Can you work these out from the model? Positions are in its coordinate system, mm. Face numbers are marked on the shaded views. A direction names the side the tool comes from. Give positions to 0.01 mm unless a question says otherwise; leave off trailing zeros. Loops run counter-clockwise (first coordinate to the right, second up) from the corner with the lowest first, then second, coordinate; pieces in that order, holes last. Notation, with made-up numbers: (-33.5, 79) -> (-11.5, 79) arc R30 ccw to (-11.5, 102) -> close; hole circle Ø9 at (63.5, 49). An arc over 180 degrees is marked (long way). One line per question, with ' | ' between items.
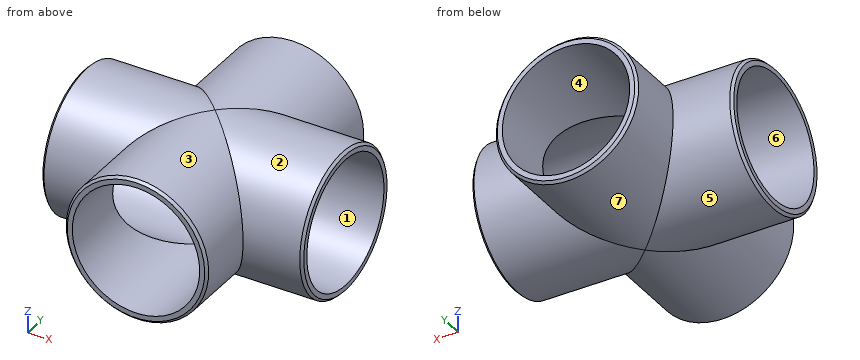
from build123d import *

# Parameters (mm, degrees)
RUNROUTE_R             = 57.15
RUNEXTRUDE_DEPTH       = 104.648
OUTLETROUTE_R          = 57.15
OUTLETEXTRUDE_DEPTH    = 104.648
CROSSSHELL_START       = -104.648
CROSSSHELL_OUTLINE_R   = 51.1302
CROSSSHELL_DEPTH       = 209.296
CROSSSHELL_2_OUTLINE_R = 51.1302
CROSSSHELL_2_DEPTH     = 209.296
CROSSCHAMFER_SIZE      = 2.0066


with BuildPart() as part:
    # RunRoute → RunExtrude (new body)
    with BuildSketch(Plane(origin=(0, 0, 0), x_dir=(0, 0, -1), z_dir=(1, 0, 0))):
        Circle(RUNROUTE_R)
    runextrude = extrude(amount=RUNEXTRUDE_DEPTH)

    # RunExtrudeMirror: RunExtrude across plane
    add(runextrude.mirror(Plane(origin=(0, 0, 0), x_dir=(0, 0, 1), z_dir=(1, 0, 0))))

    # OutletRoute → OutletExtrude (add)
    with BuildSketch(Plane(origin=(0, 0, 0), x_dir=(1, 0, 0), z_dir=(0, 1, 0))):
        with Locations(Location((0, 0, 0), (0, 0, 270))):
            Circle(OUTLETROUTE_R)
    outletextrude = extrude(amount=OUTLETEXTRUDE_DEPTH)

    # OutletExtrudeMirror: OutletExtrude across plane
    add(outletextrude.mirror(Plane.ZX))

    # CrossShell: read off the stored shape, not the designer's step
    # CrossShell outline → CrossShell (cut)
    with BuildSketch(Plane.YZ.offset(CROSSSHELL_START)):
        Circle(CROSSSHELL_OUTLINE_R)
    extrude(amount=CROSSSHELL_DEPTH, mode=Mode.SUBTRACT)

    # CrossShell 2 outline → CrossShell 2 (cut)
    with BuildSketch(Plane(origin=(0, 0, 0), x_dir=(1, 0, 0), z_dir=(0, 1, 0)).offset(CROSSSHELL_START)):
        Circle(CROSSSHELL_2_OUTLINE_R)
    extrude(amount=CROSSSHELL_2_DEPTH, mode=Mode.SUBTRACT)

    # CrossChamfer
    crosschamfer_edges = [part.edges().sort_by_distance(p)[0] for p in [
        (0, -104.648, -57.15),
        (104.648, 0, 57.15),
        (-104.648, 0, 57.15),
        (0, 104.648, -57.15),
    ]]
    chamfer(crosschamfer_edges, length=CROSSCHAMFER_SIZE)


solid = part.part
Q1. If we section it at B-B (y = 67.5): Write out the boundary of the cut face in (x, z).
Entries:
outline: circle Ø114.3 at (0, 0); hole circle Ø102.26 at (0, 0)
Q2. If we section it at A-A (z = 0): State how many separate pieces and enclosed holes the cut face has, plus the area to 3 significant figures.
Entries:
separate pieces: 4 | enclosed holes: 0 | area: 2,420 mm²
Q3. For pin 1 Ø6 at (x, y) = (78.5, -8) entering from -Z; pin 2 Ø8 at (x, z) = (70.5, 14) entering from -Y; pin 3 Ø6 at (x, y) = (61, 52) entering from -Z, each with a flat end and sliding along its axis, tell me the tip position at first contact or that it passes through.
Entries:
pin 1: z = -56.93 | pin 2: y = -56.27 | pin 3: z = -29.41
Q4. On a 3-axis mill with a long thin cutter (end or side, diameter ignored), from which of +Z, -Z, +X, -X, +Y, -Y can I reach the whole of each face in a straight line? I mean the marked faces 3, 4, 5, 6 and 7. Say none if no direction works.
Entries:
face 3: -Y | face 4: +Y, -Y | face 5: -X | face 6: +X, -X | face 7: +Y
Q5. If I drill on probe 1 along X at (y, z) = (-65, 0); probe 2 along Z at (x, y) = (-28.5, -23.5), over which ranges is the centre line in solid material (lowest first)? Write a range as from..to.
Entries:
probe 1: -57.15..-51.13, 51.13..57.15 | probe 2: -52.09..-45.41, 45.41..52.09
Q6. If we mould it in two halves opening along Y, with no side actions, what happens to the marked faces 1 and 2? For each: pulls with the +Y half, pulls with the -Y half, needs draft (parallel to the pull), parting line crosses it, or undercut.
Entries:
face 1: undercut | face 2: parting line crosses it
